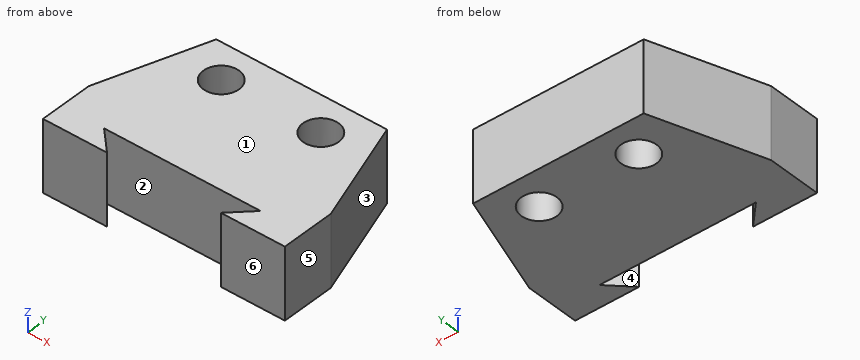
from build123d import *

# Parameters (mm, degrees)
SKETCH1_R           = 5
BOSS_EXTRUDE1_DEPTH = 10


with BuildPart() as part:
    # Sketch1 → Boss-Extrude1 (new, symmetric)
    with BuildSketch(Plane.XY):
        Polygon((-24, 39), (24, 39), (34, 9), (34, 0), (34, -6), (16, -6), (22, 0), (-22, 0), (-16, -6), (-34, -6), (-34, 0), (-34, 9), align=None)
        with Locations((-14, 29)):
            Circle(SKETCH1_R, mode=Mode.SUBTRACT)
        with Locations((14, 29)):
            Circle(SKETCH1_R, mode=Mode.SUBTRACT)
    extrude(amount=BOSS_EXTRUDE1_DEPTH, both=True)


solid = part.part
For this review, take the finished solid that the model builds, in its own axes (mm). Face numbers are marked on the shaded views. A direction names the side the tool comes from. Coordinates: 2 decimals unless noted, no trailing zeros. Loops run counter-clockwise (first coordinate to the right, second up) from the corner with the lowest first, then second, coordinate; pieces in that order, holes last. Notation, with made-up numbers: (2, 72.25) - (39, 72.25) arc R13 cw to (39, 77.25) - close; hole circle Ø11 at (52.5, 15.25). An arc over 180 degrees is marked (long way). Return JSON: item names as keys, results as strings.
Item 1: For line 1 (X direction, y = 28.5, z = -2.75); line 2 (Y direction, x = 14, z = 4.5); line 3 (Y direction, x = 6.5, z = 9), list the stretches that pass through material, from the lowest coordinate up.
Determined:
{"line 1": "x = -27.5 to -18.97, -9.03 to 9.03, 18.97 to 27.5", "line 2": "y = 0 to 24, 34 to 39", "line 3": "y = 0 to 39"}
Item 2: Take a section at D-D (y = 26). Give the boundary of the cut face in (x, z).
Determined:
{"outline": "(-28.33, -10) - (-18, -10) - (-18, 10) - (-28.33, 10) - close; (-10, -10) - (10, -10) - (10, 10) - (-10, 10) - close; (18, -10) - (28.33, -10) - (28.33, 10) - (18, 10) - close"}
Item 3: Take a section at B-B (y = -2). Give the boundary of the cut face in (x, z).
Determined:
{"outline": "(-34, -10) - (-20, -10) - (-20, 10) - (-34, 10) - close; (20, -10) - (34, -10) - (34, 10) - (20, 10) - close"}
Item 4: For the marked faces 1 and 2, list the 3-axis set-ups (+Z, -Z, +X, -X, +Y, -Y) from which the entire face can be reached by the end or side of a thin tool; tool diameter is ignored.
Determined:
{"face 1": "+Z, +X, -X, +Y, -Y", "face 2": "+Z, -Z"}
Item 5: Mouldability with a two-part tool opening along Y and no side actions: class the marked faces 3, 4, 5 and 6 as pulls with the +Y half, pulls with the -Y half, needs draft (parallel to the pull), parting line crosses it, or undercut.
Determined:
{"face 3": "pulls with the +Y half", "face 4": "undercut", "face 5": "needs draft", "face 6": "pulls with the -Y half"}
Item 6: Insertion check: pin 1 (5 mm diameter, centred on x = -7, z = 2.5, fed in from -Y); pin 2 (1 mm diameter, centred on y = 17.5, z = -2.5, fed in from -X); pin 3 (13 mm diameter, centred on x = -14, y = 29, fed in from +Z). Each pin has a flat end and moves straight along its axis. Give the tip position at first contact, or say it passes through.
Determined:
{"pin 1": "stops at y = 0", "pin 2": "stops at x = -31.33", "pin 3": "stops at z = 10"}
Item 7: Take a section at A-A (x = 20.5). Give the boundary of the cut face in (y, z), then the cut area to 3 significant figures.
Determined:
{"outline": "(-6, -10) - (-1.5, -10) - (-1.5, 10) - (-6, 10) - close; (0, -10) - (39, -10) - (39, 10) - (0, 10) - close", "area": "870 mm2"}
Item 8: Take a section at C-C (z = 2.75). Give the boundary of the cut face in (x, y), then the cut area to 3 significant figures.
Determined:
{"outline": "(-34, -6) - (-16, -6) - (-22, 0) - (22, 0) - (16, -6) - (34, -6) - (34, 9) - (24, 39) - (-24, 39) - (-34, 9) - close; hole circle Ø10 at (-14, 29); hole circle Ø10 at (14, 29)", "area": "2,370 mm2"}
